from build123d import *

# Parameters (mm, degrees)
CROQUIS1_R              = 1.5
CROQUIS1_R_2            = 2
CROQUIS1_R_3            = 1
CROQUIS1_W              = 7
CROQUIS1_H              = 45
SALIENTE_EXTRUIR2_DEPTH = 3


with BuildPart() as part:
    # Croquis1 → Saliente-Extruir2 (new body)
    with BuildSketch(Plane(origin=(0, 0, 0), x_dir=(1, 0, 0), z_dir=(0, 1, 0))):
        Polygon((-75, -75), (-75, -65), (-72, -65), (-72, -55), (-75, -55), (-75, -45), (-72, -45), (-72, -35), (-75, -35), (-75, -25), (-72, -25), (-72, -15), (-75, -15), (-75, -5), (-72, -5), (-72, 5), (-75, 5), (-75, 15), (-72, 15), (-72, 25), (-75, 25), (-75, 35), (-72, 35), (-72, 45), (-75, 45), (-75, 55), (-72, 55), (-72, 65), (-75, 65), (-75, 75), (-65, 75), (-65, 72), (-55, 72), (-55, 47), (-45, 47), (-45, 52), (15, 52), (15, 72), (25, 72), (25, 75), (35, 75), (35, 72), (45, 72), (45, 75), (55, 75), (55, 72), (65, 72), (65, 75), (75, 75), (75, 65), (72, 65), (72, 55), (75, 55), (75, 45), (72, 45), (72, 35), (75, 35), (75, 25), (72, 25), (72, 15), (75, 15), (75, 5), (72, 5), (72, -5), (75, -5), (75, -15), (72, -15), (72, -25), (75, -25), (75, -35), (72, -35), (72, -45), (75, -45), (75, -55), (72, -55), (72, -65), (75, -65), (75, -75), (65, -75), (65, -72), (55, -72), (55, -75), (45, -75), (45, -72), (35, -72), (35, -75), (25, -75), (25, -72), (15, -72), (15, -52), (-45, -52), (-45, -47), (-55, -47), (-55, -72), (-65, -72), (-65, -75), align=None)
        with Locations(Location((65, 12.5, 0), (0, 0, 270))):
            Circle(CROQUIS1_R, mode=Mode.SUBTRACT)
        with Locations(Location((65, -12.5, 0), (0, 0, 90))):
            Circle(CROQUIS1_R, mode=Mode.SUBTRACT)
        with Locations(Location((66, 66, 0), (0, 0, 270))):
            Circle(CROQUIS1_R_2, mode=Mode.SUBTRACT)
        with Locations(Location((34, 66, 0), (0, 0, 270))):
            Circle(CROQUIS1_R_2, mode=Mode.SUBTRACT)
        with Locations(Location((66, 46, 0), (0, 0, 270))):
            Circle(CROQUIS1_R_2, mode=Mode.SUBTRACT)
        with Locations(Location((34, 46, 0), (0, 0, 270))):
            Circle(CROQUIS1_R_2, mode=Mode.SUBTRACT)
        with Locations(Location((66, -46, 0), (0, 0, 90))):
            Circle(CROQUIS1_R_2, mode=Mode.SUBTRACT)
        with Locations(Location((34, -46, 0), (0, 0, 90))):
            Circle(CROQUIS1_R_2, mode=Mode.SUBTRACT)
        with Locations(Location((66, -66, 0), (0, 0, 90))):
            Circle(CROQUIS1_R_2, mode=Mode.SUBTRACT)
        with Locations(Location((34, -66, 0), (0, 0, 90))):
            Circle(CROQUIS1_R_2, mode=Mode.SUBTRACT)
        with Locations(Location((-66, 16, 0), (0, 0, 270))):
            Circle(CROQUIS1_R_2, mode=Mode.SUBTRACT)
        with Locations(Location((-66, -16, 0), (0, 0, 270))):
            Circle(CROQUIS1_R_2, mode=Mode.SUBTRACT)
        with Locations(Location((-46, 16, 0), (0, 0, 270))):
            Circle(CROQUIS1_R_2, mode=Mode.SUBTRACT)
        with Locations(Location((-46, -16, 0), (0, 0, 270))):
            Circle(CROQUIS1_R_2, mode=Mode.SUBTRACT)
        with Locations(Location((46.1, 34.675, 0), (0, 0, 270))):
            Circle(CROQUIS1_R_3, mode=Mode.SUBTRACT)
        with Locations(Location((46.1, -34.675, 0), (0, 0, 90))):
            Circle(CROQUIS1_R_3, mode=Mode.SUBTRACT)
        with Locations(Location((46.1, 21.475, 0), (0, 0, 270))):
            Circle(CROQUIS1_R_3, mode=Mode.SUBTRACT)
        Polygon((59.1, -10.5), (59.1, -7.5), (59.1, 7.5), (59.1, 10.5), (62.1, 10.5), (62.1, -10.5), align=None, mode=Mode.SUBTRACT)
        with Locations((47.6, -7.175)):
            Rectangle(CROQUIS1_W, CROQUIS1_H, mode=Mode.SUBTRACT)
    extrude(amount=SALIENTE_EXTRUIR2_DEPTH)


solid = part.part
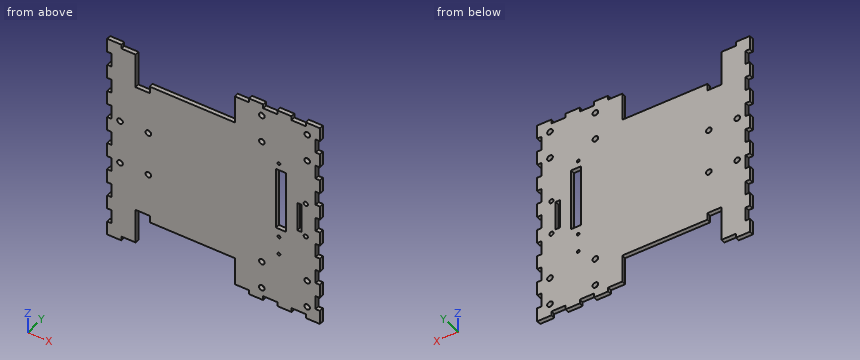
Can you work these out from the model? Positions are in its coordinate system, mm. Coordinates: 2 decimals unless noted, no trailing zeros. Write each loop counter-clockwise with the first axis right and the second up, starting at its lowest first coordinate (ties: lowest second). Pieces come first, ordered by that corner, then holes.
Q1. For P1, Ø2.5, axis at x = 66, z = 66, coming from the -Y side; P2, Ø1.5, axis at y = 1, z = 18, coming from the +X side; P3, Ø5, axis at x = 65, z = -12.5, coming from the -Y side; P4, Ø1.5, axis at x = -60.5, y = 1.5, coming from the +Z side, each with a flat end and sliding along its axis, tell me the tip position at first contact or that it passes through.
Results found:
P1: passes through
P2: stops at x = 72
P3: stops at y = 0
P4: stops at z = 72
Q2. Imagine slicing it at B-B, the plane x = -25. List the corners of the cut face in (y, z) for me, plus the area to 3 significant figures.
Results found:
outline: (0, -52) - (3, -52) - (3, 52) - (0, 52) - close
area: 312 mm2
Q3. Imagine slicing it at A-A, the plane y = 1.9. Count the separate pieces of the cut face and the enclosed holes in it, plus the area to 3 significant figures.
Results found:
separate pieces: 1
enclosed holes: 19
area: 18,000 mm2
Q4. Please list where these lines run through material, in increasing order: L1, parallel to X at y = 0.7, z = -10; L2, parallel to X at y = 2.2, z = 66; L3, parallel to X at y = 1.6, z = -16.
Results found:
L1: x = -75 to 44.1, 51.1 to 59.1, 62.1 to 75
L2: x = -75 to -55, 15 to 32, 36 to 64, 68 to 75
L3: x = -72 to -68, -64 to -48, -44 to 72
